from build123d import *

# Parameters (mm, degrees)
SKETCH1_W               = 30.5
SKETCH1_H               = 21.5
SKETCH1_W_2             = 26.5
SKETCH1_H_2             = 17.5
BOSS_EXTRUDE1_DEPTH     = 46.5
FILLET1_R               = 2
SKETCH2_W               = 2.094102849
SKETCH2_H               = 5.748513101
BOSS_EXTRUDE2_DEPTH     = 5
CUT_EXTRUDE1_START      = -3.094102849
SKETCH3_R               = 1.525
CUT_EXTRUDE1_DEPTH      = 23.5
MIRROR4_COPY_1_SKETCH_W = 2.094102849
MIRROR4_COPY_1_SKETCH_H = 5.748513101
MIRROR4_COPY_1_DEPTH    = 5
MIRROR4_START           = -3.094102849
MIRROR4_COPY_2_SKETCH_R = 1.525
MIRROR4_COPY_2_DEPTH    = 23.5
FILLET2_R               = 2
BOSS_EXTRUDE4_DEPTH     = 2
CUT_EXTRUDE2_DEPTH      = 6
CUT_EXTRUDE2_DEPTH_BACK = 36.5


with BuildPart() as part:
    # Sketch1 → Boss-Extrude1 (new body)
    with BuildSketch(Plane(origin=(0, 0, 0), x_dir=(1, 0, 0), z_dir=(0, 1, 0))):
        Rectangle(SKETCH1_W, SKETCH1_H)
        Rectangle(SKETCH1_W_2, SKETCH1_H_2, mode=Mode.SUBTRACT)
    extrude(amount=BOSS_EXTRUDE1_DEPTH)

    # Fillet1
    fillet1_edges = [part.edges().sort_by_distance(p)[0] for p in [
        (-15.25, 23.25, 10.75),
        (15.25, 23.25, 10.75),
    ]]
    fillet(fillet1_edges, radius=FILLET1_R)

    # Sketch2 → Boss-Extrude2 (add)
    with BuildSketch(Plane.ZY.offset(15.25)):
        with Locations((-9.702948576, 2.874256551)):
            Rectangle(SKETCH2_W, SKETCH2_H)
    boss_extrude2 = extrude(amount=BOSS_EXTRUDE2_DEPTH)

    # Sketch3 → Cut-Extrude1 (cut)
    with BuildSketch(Plane.XY.offset(-8.655897151).offset(CUT_EXTRUDE1_START)):
        with Locations((-17.75, 2.874256551)):
            Circle(SKETCH3_R)
    cut_extrude1 = extrude(amount=CUT_EXTRUDE1_DEPTH, mode=Mode.SUBTRACT)

    # Mirror3: Boss-Extrude2, Cut-Extrude1 across plane
    add(boss_extrude2.mirror(Plane.ZX.offset(23.25)))
    add(cut_extrude1.mirror(Plane.ZX.offset(23.25)), mode=Mode.SUBTRACT)

    # Mirror4: Boss-Extrude2, Cut-Extrude1 across plane
    add(boss_extrude2.mirror(Plane(origin=(0, 0, 0), x_dir=(0, 0, 1), z_dir=(1, 0, 0))))
    add(cut_extrude1.mirror(Plane(origin=(0, 0, 0), x_dir=(0, 0, 1), z_dir=(1, 0, 0))), mode=Mode.SUBTRACT)

    # Mirror4 copy 1 sketch → Mirror4 copy 1 (add)
    with BuildSketch(Plane(origin=(15.25, 46.5, 0), x_dir=(0, 0, 1), z_dir=(1, 0, 0))):
        with Locations((-9.702948576, 2.874256551)):
            Rectangle(MIRROR4_COPY_1_SKETCH_W, MIRROR4_COPY_1_SKETCH_H)
    extrude(amount=MIRROR4_COPY_1_DEPTH)

    # Mirror4 copy 2 sketch → Mirror4 copy 2 (cut)
    with BuildSketch(Plane(origin=(0, 46.5, -8.655897151), x_dir=(-1, 0, 0), z_dir=(0, 0, 1)).offset(MIRROR4_START)):
        with Locations((-17.75, 2.874256551)):
            Circle(MIRROR4_COPY_2_SKETCH_R)
    extrude(amount=MIRROR4_COPY_2_DEPTH, mode=Mode.SUBTRACT)

    # Fillet2
    fillet2_edges = [part.edges().sort_by_distance(p)[0] for p in [
        (-20.25, 0, -9.702948576),
        (-20.25, 5.748513101, -9.702948576),
        (-20.25, 40.751486899, -9.702948576),
        (-20.25, 46.5, -9.702948576),
        (20.25, 46.5, -9.702948576),
        (20.25, 40.751486899, -9.702948576),
        (20.25, 5.748513101, -9.702948576),
        (20.25, 0, -9.702948576),
    ]]
    fillet(fillet2_edges, radius=FILLET2_R)

    # Sketch4 → Boss-Extrude4 (add)
    with BuildSketch(Plane.XZ):
        with BuildLine():
            Line((15.25, -10.75), (-15.25, -10.75))
            Line((-15.25, -10.75), (-15.25, 8.75))
            ThreePointArc((-15.25, 8.75), (-14.664213562, 10.164213562), (-13.25, 10.75))
            Line((-13.25, 10.75), (13.25, 10.75))
            ThreePointArc((13.25, 10.75), (14.664213562, 10.164213562), (15.25, 8.75))
            Line((15.25, 8.75), (15.25, -10.75))
        make_face()
    extrude(amount=BOSS_EXTRUDE4_DEPTH)

    # Sketch6 → Cut-Extrude2 (cut, two sides)
    with BuildSketch(Plane.ZY.offset(15.25)) as cut_extrude2_sk:
        Polygon((-5.75, 22.25), (4.25, 16.476497308), (4.25, 28.023502692), align=None)
        Polygon((-5.75, 38.726497308), (4.25, 32.952994616), (4.25, 44.5), align=None)
        Polygon((-5.75, 5.773502692), (4.25, 0), (4.25, 11.547005384), align=None)
        Polygon((4.25, 30.439180122), (-5.75, 36.212682814), (-5.75, 24.66567743), align=None)
        Polygon((-5.75, 19.83432257), (4.25, 14.060819878), (-5.75, 8.287317186), align=None)
    extrude(amount=CUT_EXTRUDE2_DEPTH, mode=Mode.SUBTRACT)
    extrude(cut_extrude2_sk.sketch, amount=-CUT_EXTRUDE2_DEPTH_BACK, mode=Mode.SUBTRACT)


solid = part.part
The model under review builds one solid part; all positions refer to its coordinate system, in mm. A direction names the side the tool comes from. Round coordinates to 2 decimals unless told otherwise and drop trailing zeros. Loops run counter-clockwise (first coordinate to the right, second up) from the corner with the lowest first, then second, coordinate; pieces in that order, holes last. Notation, with made-up numbers: M 19,-26.75 L 44,-26.75 A12 ccw 44,-10.75 Z; hole C -2.75,34 d2. An arc over 180 degrees is marked long. Answer as CSV lines item,"result". Start each with the question number.
Item 1: Consider section A-A (x = 4.5). Write out the cut boundary in (y, z), then the cut area to 3 significant figures.
Item 2: For faces 4 (the face through (14.24, 16.99, -0.82)), 5 (the face through (-19.68, 41.353, -9.688)), 6 (the face through (13.25, 28, 2)), list the 3-axis set-ups (+Z, -Z, +X, -X, +Y, -Y) from which the entire face can be reached by the end or side of a thin tool; tool diameter is ignored.
Item 3: Consider section B-B (z = 7). Write out the cut boundary in (x, y), then the cut area to 3 significant figures.
Item 4: Insertion check: P1, Ø5, axis at y = 16.5, z = 0.5, coming from the +X side; P2, Ø1.5, axis at x = -17.5, y = 3, coming from the +Z side; P3, Ø4, axis at y = 8, z = 6.5, coming from the -X side; P4, Ø1, axis at x = -11, z = -8, coming from the +Y side. Each pin has a flat end and moves straight along its axis. Give the tip position at first contact, or say it passes through.
Item 5: Wall thickness on line 1 (Y direction, x = 17.75, z = -9.45); line 2 (Z direction, x = 14.5, y = 10); line 3 (Z direction, x = -6, y = 7.5): over which ranges is each line inside the solid? List them lowest first. Write a range as [from, to].
Item 6: Mouldability with a two-part tool opening along Y and no side actions: class faces 1 (the face through (0, -2, 0)), 2 (the face through (20.25, 3, -10)), 3 (the face through (-14.26, 8.7, -0.68)) as released by +Y, released by -Y, zero draft, split by the parting line, or undercut.
Item 7: Consider section C-C (y = 29.5). Write out the cut boundary in (x, z), then the cut area to 3 significant figures.
Answer:
1,outline,"M -2,-10.75 L 46.5,-10.75 L 46.5,-8.75 L 0,-8.75 L 0,8.75 L 46.5,8.75 L 46.5,10.75 L -2,10.75 Z"
1,area,"229 mm^2"
2,face 4,"+X, -X"
2,face 5,"+Z, -Z, -X"
2,face 6,"+Y"
3,outline,"M -15.25,-2 L 15.25,-2 L 15.25,46.5 L 13.25,46.5 L 13.25,0 L -13.25,0 L -13.25,46.5 L -15.25,46.5 Z"
3,area,"247 mm^2"
4,P1,"stops at x = 15.25"
4,P2,"passes through"
4,P3,"stops at x = -15.25"
4,P4,"stops at y = 0"
5,line 1,"y = [0, 1.35], [4.4, 5.75], [40.75, 42.1], [45.15, 46.5]"
5,line 2,"z = [-10.75, -5.75], [-2.78, 1.57], [4.25, 10.31]"
5,line 3,"z = [-10.75, -8.75], [8.75, 10.75]"
6,face 1,"released by -Y"
6,face 2,"zero draft"
6,face 3,"undercut"
7,outline,"M -15.25,-10.75 L 15.25,-10.75 L 15.25,-5.75 L 13.25,-5.75 L 13.25,-8.75 L -13.25,-8.75 L -13.25,-5.75 L -15.25,-5.75 Z; M -15.25,2.62 L -13.25,2.62 L -13.25,8.75 L 13.25,8.75 L 13.25,2.62 L 15.25,2.62 L 15.25,8.75 A2 ccw 13.25,10.75 L -13.25,10.75 A2 ccw -15.25,8.75 Z"
7,area,"157 mm^2"
